Autodesk Inventor part; units mm, degrees
ref_plane "YZ Plane" through (0, 0, 0) normal (1, 0, 0) x (0, 1, 0)
ref_plane "XZ Plane" through (0, 0, 0) normal (0, 1, 0) x (-1, 0, 0)
ref_plane "XY Plane" through (0, 0, 0) normal (0, 0, 1) x (1, 0, 0)
sketch "Sketch1" plane through (0, 0, 0) normal (0, 0, 1) x (1, 0, 0)
  circle A0 centre (-43.9941, 0) radius 9.525
  circle A1 centre (43.9941, 0) radius 6.35
  line L0 (43.9941, 0) -> (-43.9941, 0) construction
  line L1 (43.9941, 12.7) -> (-43.9941, 12.7)
  line L2 (-43.9941, -12.7) -> (43.9941, -12.7)
  arc A2 (43.9941, -12.7) -> (43.9941, 12.7) centre (43.9941, 0) ccw
  arc A3 (-43.9941, 12.7) -> (-43.9941, -12.7) centre (-43.9941, 0) ccw
  point P0 (0, 0)
  point P1 (0, 0)
  dimension "d10" = 12.7
  dimension "d11" = 19.05
  dimension "d12" = 87.9881
  dimension "d13" = 12.7
sketch "Sketch3" plane through (0, 0, 0) normal (0, 0, 1) x (1, 0, 0)
  line L0 (-44.9008, 0) -> (44.9008, 0) construction
  line L1 (-44.9008, -12.7) -> (44.9008, -12.7)
  line L2 (44.9008, 12.7) -> (-44.9008, 12.7)
  arc A0 (-44.9008, 12.7) -> (-44.9008, -12.7) centre (-44.9008, 0) ccw
  arc A1 (44.9008, -12.7) -> (44.9008, 12.7) centre (44.9008, 0) ccw
  circle A2 centre (-44.9008, 0) radius 6.35
  point P0 (0, 0)
  dimension "d23" = 44.9008
  dimension "d24" = 25.4
  dimension "d25" = 12.7
extrude "Extrusion4" add sketch "Sketch3" against normal blind 8.4667
sketch "Sketch4" plane through (0, 0, -8.4667) normal (0, 0, -1) x (-1, 0, 0)
  circle A0 centre (-44.9008, 0) radius 6.35
  arc A1 (-44.9008, 12.7) -> (-44.9008, -12.7) centre (-44.9008, 0) ccw
  point P0 (0, 0)
  dimension "d28" = 12.7
extrude "Extrusion5" cut sketch "Sketch4" against normal through all
sketch "Sketch5" plane through (0, 0, -8.4667) normal (0, 0, -1) x (-1, 0, 0)
  circle A0 centre (44.9008, 0) radius 6.35
  line L0 (61.8342, 29.3294) -> (78.7675, 0)
  line L1 (78.7675, 0) -> (61.8342, -29.3294)
  line L2 (61.8342, -29.3294) -> (27.9675, -29.3294)
  line L3 (27.9675, -29.3294) -> (11.0342, 0)
  line L4 (11.0342, 0) -> (27.9675, 29.3294)
  line L5 (27.9675, 29.3294) -> (61.8342, 29.3294)
  line L6 (-44.9008, 12.7) -> (44.9008, 12.7)
  point P0 (0, 0)
  dimension "d31" = 33.8667
extrude "Extrusion6" add sketch "Sketch5" against normal up to surface (8.4667 mm away)
sketch "Sketch7" plane through (0, 0, -8.4667) normal (0, 0, -1) x (-1, 0, 0)
  circle A0 centre (-44.9008, 0) radius 6.35
  circle A1 centre (-44.9008, 0) radius 12.7
  line L0 (-44.9008, -12.7) -> (18.3665, -12.7)
  line L1 (-66.8979, 0) -> (-55.8994, 19.05)
  line L2 (-55.8994, 19.05) -> (-33.9023, 19.05)
  line L3 (-33.9023, 19.05) -> (-22.9038, 0)
  line L4 (-22.9038, 0) -> (-33.9023, -19.05)
  line L5 (-33.9023, -19.05) -> (-55.8994, -19.05)
  line L6 (-55.8994, -19.05) -> (-66.8979, 0)
  point P0 (0, 0)
  point P1 (5.3062, -12.7)
  dimension "d48" = 38.1
extrude "Extrusion8" add sketch "Sketch7" against normal up to surface (8.4667 mm away) contours L1 L2 L3 L4 L5 L6
sketch "Sketch12" plane through (0, 0, -8.4667) normal (0, 0, -1) x (-1, 0, 0)
  circle A0 centre (44.9008, 0) radius 6.35
  circle A1 centre (44.9008, 0) radius 8.4667
  point P0 (0, 0)
  dimension "d73" = 16.9333
extrude "Extrusion12" add sketch "Sketch12" against normal blind 25.4 contours A0 | A1
sketch "Sketch13" plane through (-44.9008, 0, 16.9333) normal (0, 0, 1) x (1, 0, 0)
  circle A0 centre (0, 0) radius 8.4667
  circle A1 centre (0, 0) radius 8.4667
  circle A2 centre (0, 0) radius 5.6444
  point P0 (44.9008, 0)
  dimension "d76" = 11.2889
extrude "Extrusion13" cut sketch "Sketch13" against normal blind 11.2889 draft -10 contours A2
sketch "Sketch14" plane through (0, 0, -8.4667) normal (0, 0, -1) x (-1, 0, 0)
  circle A0 centre (-44.9008, 0) radius 6.35
  circle A1 centre (-44.9008, 0) radius 6.35
  point P0 (0, 0)
  dimension "d79" = 12.7
extrude "Extrusion14" add sketch "Sketch14" against normal blind 25.4
sketch "Sketch15" plane through (44.9008, 0, 16.9333) normal (0, 0, 1) x (1, 0, 0)
  circle A0 centre (0, 0) radius 6.35
  circle A1 centre (0, 0) radius 4.2333
  point P0 (-44.9008, 0)
  dimension "d82" = 8.4667
extrude "Extrusion15" cut sketch "Sketch15" against normal blind 11.2889 draft -10 contours A1
properties part number "Frame" material "ABS Plastic"
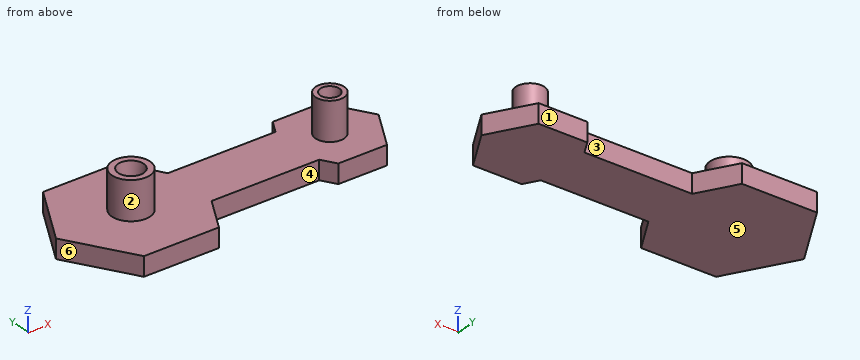
Here's how the part is built. I have some questions about the finished solid (model axes, mm). Face numbers are marked on the shaded views. A direction names the side the tool comes from. Give positions to 0.01 mm unless a question says otherwise; leave off trailing zeros. Order: outer loops, then holes, each group sorted by start corner. A loop starts at its lowest first (then second) coordinate and runs counter-clockwise, first axis right, second up. Notation, with made-up numbers: (9.5, 29) -> (57.5, 29) arc R27 ccw to (57.5, 56) -> close; hole circle Ø3 at (63, -8.75). An arc over 180 degrees is marked (long way). One line per item, written item: value. Start each with the question number.
1. For the marked faces 1, 2 and 3, which set-ups out of +Z, -Z, +X, -X, +Y, -Y let a thin tool reach every point of the face, with its end or its side?
2. We'd pull the mould along X, two halves only. Please class the marked faces 4, 5 and 6: released by +X, released by -X, zero draft, split by the parting line, or undercut.
3. I need wall thicknesses on probe 1 along Y at (x, z) = (3, -6.5); probe 2 along Z at (x, y) = (46.5, -13.5); probe 3 along X at (y, z) = (19, -7). Which ranges of each line are inside material? Lowest first, please. Write a range as from..to.
4. Imagine slicing it at B-B, the plane y = -14. List the corners of the cut face in (x, z) for me, plus the area to 3 significant figures.
5. Will these pins go through, and if not, where does the flat tip stop? pin 1 Ø4 at (x, y) = (-36.5, -10) entering from +Z; pin 2 Ø5 at (y, z) = (-0.5, 11) entering from +X; pin 3 Ø1.5 at (x, z) = (-3, 2.5) entering from -Y; pin 4 Ø3 at (x, z) = (51, 1) entering from +Y.
6. Imagine slicing it at D-D, the plane y = 21. List the corners of the cut face in (x, z) for me, plus the area to 3 significant figures.
7. Imagine slicing it at A-A, the plane z = 8.25. List the corners of the cut face in (x, y) for me.
8. Imagine slicing it at C-C, the plane z = -2. List the corners of the cut face in (x, y) for me, plus the area to 3 significant figures.
Values follow:
1. face 1: +Z, -Z, +X, +Y
1. face 2: +Z
1. face 3: +Z, -Z, +Y
2. face 4: undercut
2. face 5: zero draft
2. face 6: released by -X
3. probe 1: y = -12.7..12.7
3. probe 2: z = -8.47..0
3. probe 3: x = -67.8..-22, 33.87..55.93
4. outline: (-70.68, -8.47) -> (-19.12, -8.47) -> (-19.12, 0) -> (-70.68, 0) -> close; (30.99, -8.47) -> (58.82, -8.47) -> (58.82, 0) -> (30.99, 0) -> close
4. area: 672 mm2
5. pin 1: stops at z = 0
5. pin 2: stops at x = 51.25
5. pin 3: passes through
5. pin 4: stops at y = 19.05
6. outline: (-66.64, -8.47) -> (-23.16, -8.47) -> (-23.16, 0) -> (-66.64, 0) -> close
6. area: 368 mm2
7. outline: circle Ø16.93 at (-44.9, 0); circle Ø12.7 at (44.9, 0); hole circle Ø8.23 at (-44.9, 0); hole circle Ø5.4 at (44.9, 0)
8. outline: (-78.77, 0) -> (-61.83, -29.33) -> (-27.97, -29.33) -> (-18.37, -12.7) -> (30.24, -12.7) -> (33.9, -19.05) -> (55.9, -19.05) -> (66.9, 0) -> (55.9, 19.05) -> (33.9, 19.05) -> (30.24, 12.7) -> (-18.37, 12.7) -> (-27.97, 29.33) -> (-61.83, 29.33) -> close
8. area: 5,290 mm2
